Geometry: see drawing. Coordinates: mm, zero at the bounding-box minimum. Round coordinates to 2 decimals unless told otherwise and drop trailing zeros. Order: outer loops, then holes, each group sorted by start corner. A loop starts at its lowest first (then second) coordinate and runs counter-clockwise, first axis right, second up. Notation, with made-up numbers: (-32.75, 24) - (12.25, 24) arc R4 cw to (12.25, 29) - close; hole circle Ø8 at (66.5, 72). An arc over 180 degrees is marked (long way). Put each result on its own line as item: value. Start each with the question number.
1) Line query: probe 1 along Y at (x, z) = (169, 7.25); probe 2 along X at (y, z) = (73, 4.5); probe 3 along Z at (x, y) = (62, 44.5). Output: solid intervals per line, ascending. Write a range as [from, to].
2) Contact query for a flat-ended pin moving along its axis: P1, Ø16.5, axis at x = 165, y = 39.5, coming from the +Z side. Output: stop coordinate, or through.
3) Mould query, pull axis X, two halves, no side actions, for the marked faces 1 and 2. Classes: +X half, -X half, draft (parallel to the pull), parting line (faces both ways), or undercut.
4) Section C-C on y = 33. Output: boundary loops of the cut face in (x, z).
5) Section B-B on x = 174. Output: boundary loops of the cut face in (y, z).
6) Section A-A on z = 3.5. Output: boundary loops of the cut face in (x, y).
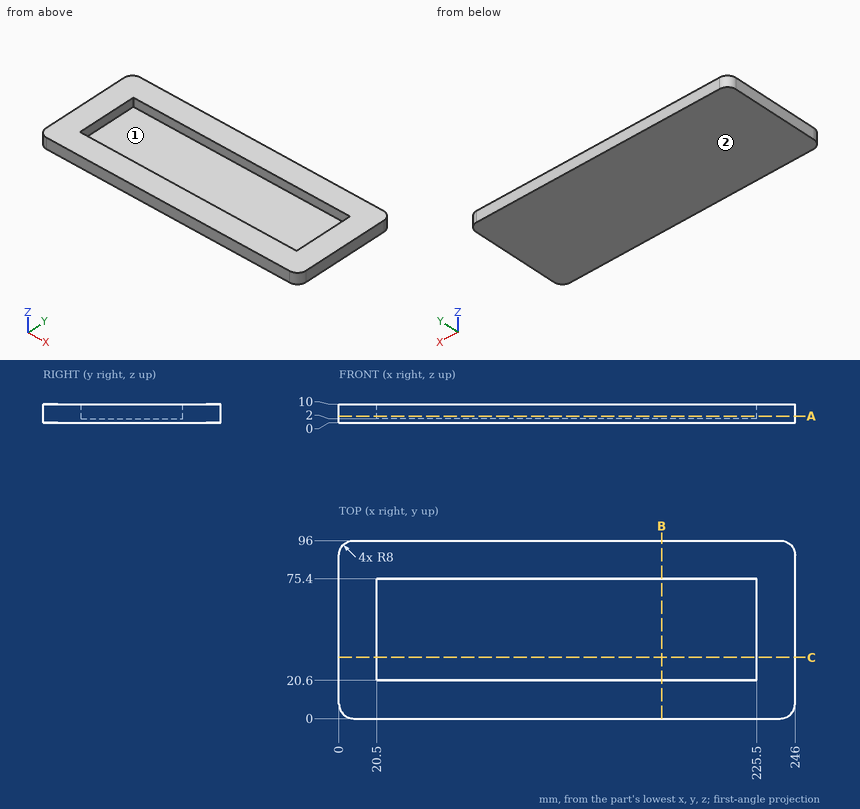
Answer sheet:
1. probe 1: [0, 20.6], [75.4, 96]
1. probe 2: [0, 20.5], [225.5, 246]
1. probe 3: [0, 2]
2. P1: z = 2
3. face 1: undercut
3. face 2: draft
4. outline: (0, 0) - (246, 0) - (246, 10) - (225.5, 10) - (225.5, 2) - (20.5, 2) - (20.5, 10) - (0, 10) - close
5. outline: (0, 0) - (96, 0) - (96, 10) - (75.4, 10) - (75.4, 2) - (20.6, 2) - (20.6, 10) - (0, 10) - close
6. outline: (0, 8) arc R8 ccw to (8, 0) - (238, 0) arc R8 ccw to (246, 8) - (246, 88) arc R8 ccw to (238, 96) - (8, 96) arc R8 ccw to (0, 88) - close; hole (20.5, 20.6) - (225.5, 20.6) - (225.5, 75.4) - (20.5, 75.4) - close
